Could you check a few things on this model? Use its own coordinates, in mm. A direction names the side the tool comes from. Round coordinates to 2 decimals unless told otherwise and drop trailing zeros. Loops run counter-clockwise (first coordinate to the right, second up) from the corner with the lowest first, then second, coordinate; pieces in that order, holes last. Notation, with made-up numbers: M 25,-34.75 L 67,-34.75 A28 cw 67,-5.75 Z; hole C -30,39 d2. An arc over 180 degrees is marked long. Answer in a Markdown table with one row per item.
```python
from build123d import *

# Parameters (mm, degrees)
CROQUIS2_R = 2


with BuildPart() as part:
    # Barrer1: sweep along a path in Croquis1
    with BuildLine(Plane.XY) as barrer1_path:
        Line((-15, 0), (-15, 15))
        ThreePointArc((-15, 15), (-13.535533906, 18.535533906), (-10, 20))
        Line((-10, 20), (10, 20))
        ThreePointArc((10, 20), (13.535533906, 18.535533906), (15, 15))
        Line((15, 15), (15, 0))
    # Croquis2 → Barrer1 (sweep)
    with BuildSketch(Plane(origin=(0, 0, 0), x_dir=(1, 0, 0), z_dir=(0, 1, 0))):
        with Locations((-15, 0)):
            Circle(CROQUIS2_R)
    sweep(path=barrer1_path.line)


solid = part.part
```
1) I want a section at B-B, the plane y = 11.75. Please give me the cut outline in (x, z), plus the area to 3 significant figures.
Computed:
| item | result |
|---|---|
| outline | C -15,0 d4; C 15,0 d4 |
| area | 25.1 mm² |
2) I want a section at C-C, the plane x = 2. Please give me the cut outline in (y, z).
Computed:
| item | result |
|---|---|
| outline | C 20,0 d4 |
3) If we mould it in two halves opening along X, with no side actions, what happens to faces 1 (the face through (0.1, 21.6, 1.2)), 2 (the face through (15, 0, 0))? For each: released by +X, released by -X, zero draft, split by the parting line, or undercut.
Computed:
| item | result |
|---|---|
| face 1 | undercut |
| face 2 | zero draft |
4) Which directions (+Z, -Z, +X, -X, +Y, -Y) give clear straight access to the entire face, cutting with the end or side of a thin tool? Please do faces 3 (the face through (-15, 0, 0)), 4 (the face through (16.6, 7.4, 1.2)).
Computed:
| item | result |
|---|---|
| face 3 | +Z, -Z, +X, -X, -Y |
| face 4 | -Y |
5) I want a section at A-A, the plane z = 0. Please give me the cut outline in (x, y), plus the area to 3 significant figures.
Computed:
| item | result |
|---|---|
| outline | M -17,0 L -13,0 L -13,15 A3 cw -10,18 L 10,18 A3 cw 13,15 L 13,0 L 17,0 L 17,15 A7 ccw 10,22 L -10,22 A7 ccw -17,15 Z |
| area | 263 mm² |
6) I need wall thicknesses on line 1 (X direction, y = 9.5, z = 0); line 2 (X direction, y = 1.25, z = -1.2); line 3 (Y direction, x = 7, z = 0). Which ranges of each line are inside material? Lowest first, please.
Computed:
| item | result |
|---|---|
| line 1 | x = -17 to -13, 13 to 17 |
| line 2 | x = -16.6 to -13.4, 13.4 to 16.6 |
| line 3 | y = 18 to 22 |
7) Will these pins go through, and if not, where does the flat tip stop? P1, Ø8, axis at x = 1.5, y = 16, coming from the +Z side; P2, Ø2, axis at x = 10, z = -0.5, coming from the -Y side.
Computed:
| item | result |
|---|---|
| P1 | stops at z = 2 |
| P2 | stops at y = 17.85 |
